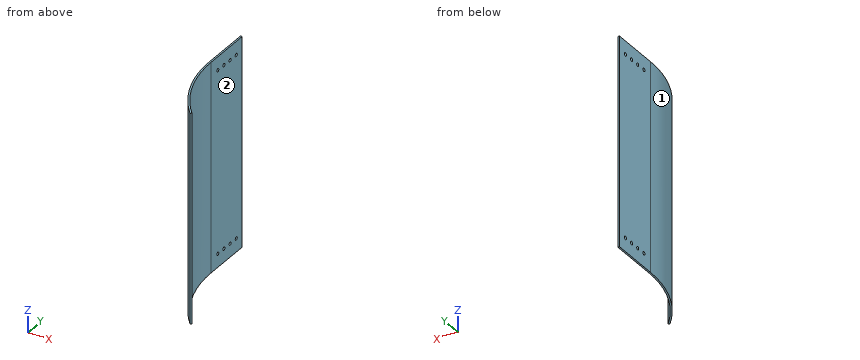
from build123d import *

# Parameters (mm, degrees)
BOSS_EXTRUDE1_DEPTH = 393.7
SKETCH2_R           = 3.175
CUT_EXTRUDE1_DEPTH  = 1537.708536769


with BuildPart() as part:
    # Sketch1 → Boss-Extrude1 (new body)
    with BuildSketch(Plane.XY):
        with BuildLine():
            Line((812.541689005, 1387.369803868), (812.541689005, 1484.270803868))
            Line((812.541689005, 1484.270803868), (815.716689005, 1484.270803868))
            Line((815.716689005, 1484.270803868), (815.716689005, 1387.369803868))
            ThreePointArc((815.716689005, 1387.369803868), (830.808178648, 1304.545262303), (874.142862637, 1232.366574946))
            Line((874.142862637, 1232.366574946), (871.757832535, 1230.270803868))
            ThreePointArc((871.757832535, 1230.270803868), (827.837227995, 1303.425406414), (812.541689005, 1387.369803868))
        make_face()
    extrude(amount=BOSS_EXTRUDE1_DEPTH)

    # Sketch2 → Cut-Extrude1 (cut, through all)
    with BuildSketch(Plane(origin=(815.716689005, 0, 0), x_dir=(0, 0, -1), z_dir=(1, 0, 0))):
        with Locations((-368.3, 1446.678803868)):
            Circle(SKETCH2_R)
        with Locations((-368.3, 1427.628803868)):
            Circle(SKETCH2_R)
        with Locations((-368.3, 1408.578803868)):
            Circle(SKETCH2_R)
        with Locations((-25.4, 1465.728803868)):
            Circle(SKETCH2_R)
        with Locations((-25.4, 1446.678803868)):
            Circle(SKETCH2_R)
        with Locations((-25.4, 1427.628803868)):
            Circle(SKETCH2_R)
        with Locations((-368.3, 1465.728803868)):
            Circle(SKETCH2_R)
        with Locations((-25.4, 1408.578803868)):
            Circle(SKETCH2_R)
    extrude(amount=-CUT_EXTRUDE1_DEPTH, mode=Mode.SUBTRACT)


solid = part.part
Work out the finished part from the listing and answer in its coordinate system (mm). Face numbers are marked on the shaded views. A direction names the side the tool comes from. Round coordinates to 2 decimals unless told otherwise and drop trailing zeros. Write each loop counter-clockwise with the first axis right and the second up, starting at its lowest first coordinate (ties: lowest second). Pieces come first, ordered by that corner, then holes.
1) Straight lines are drawn through the part: line 1 (X direction, y = 1451.5, z = 249); line 2 (X direction, y = 1370.5, z = 38); line 3 (Y direction, x = 840.5, z = 96.5). For each, find the intervals that lie inside material, in ascending order.
2) A cutting plane is placed at A-A (z = 320). Give the vertices of the cut face in (x, y).
3) A cutting plane is placed at B-B (x = 862). Give the vertices of the cut face in (y, z).
4) A tool of negligible diameter and unlimited length cuts with its end or side. For the marked faces 1 and 2, from which of +Z, -Z, +X, -X, +Y, -Y can it reach the whole face along a straight path? Write none if from no direction.
5) Given pin 1 Ø10 at (x, z) = (825, 345) entering from -Y; pin 2 Ø5 at (x, z) = (859.5, 259.5) entering from +Y; pin 3 Ø10 at (y, z) = (1425, 316) entering from +X, each flat-ended and moving along its own axis, determine where each tip first touches the part or whether it passes through.
6) A cutting plane is placed at C-C (y = 1278.5). Give the vertices of the cut face in (x, z), plus the area to 3 significant figures.
Completed:
1. line 1: x = 812.54 to 815.72
1. line 2: x = 813.14 to 816.32
1. line 3: y = 1275.45 to 1282.37
2. outline: (812.54, 1387.37) arc R238 ccw to (871.76, 1230.27) - (874.14, 1232.37) arc R234.82 cw to (815.72, 1387.37) - (815.72, 1484.27) - (812.54, 1484.27) - close
3. outline: (1242.13, 0) - (1247.39, 0) - (1247.39, 393.7) - (1242.13, 393.7) - close
4. face 1: +Z, -Z, -X, -Y
4. face 2: +Z, -Z, +X, +Y
5. pin 1: stops at y = 1297.9
5. pin 2: stops at y = 1254.39
5. pin 3: stops at x = 815.72
6. outline: (838.9, 0) - (842.48, 0) - (842.48, 393.7) - (838.9, 393.7) - close
6. area: 1,410 mm2
